from build123d import *

# Parameters (mm, degrees)
F0_W           = 304.8
F0_H           = 25.4
F1_DEPTH       = 101.6
F3_DEPTH       = 101.6
F5_D           = 10.0838
F5_CSINK_D     = 19.8374
F5_CSINK_ANGLE = 82
F7_D           = 13.49248
F8_SIZE        = 9.525
F9_SIZE        = 9.525


with BuildPart() as f1:
    # F0 (on Front) → F1 (new body, symmetric)
    with BuildSketch(Plane.XZ):
        Rectangle(F0_W, F0_H)
    extrude(amount=F1_DEPTH, both=True)

    # F2 (on Right) → F3 (join, symmetric)
    with BuildSketch(Plane.YZ):
        with BuildLine():
            Line((-82.55, 19.05), (-82.55, 12.7))
            Line((-82.55, 12.7), (-6.35, 12.7))
            Line((-6.35, 12.7), (-6.35, 88.9))
            Line((-6.35, 88.9), (-12.7, 88.9))
            ThreePointArc((-12.7, 88.9), (-14.9450640303, 87.9700640303), (-15.875, 85.725))
            Line((-15.875, 85.725), (-15.875, 28.575))
            ThreePointArc((-15.875, 28.575), (-17.7348719395, 24.0848719395), (-22.225, 22.225))
            Line((-22.225, 22.225), (-79.375, 22.225))
            ThreePointArc((-79.375, 22.225), (-81.6200640303, 21.2950640303), (-82.55, 19.05))
        make_face()
        with BuildLine():
            Line((6.35, 88.9), (6.35, 12.7))
            Line((6.35, 12.7), (82.55, 12.7))
            Line((82.55, 12.7), (82.55, 19.05))
            ThreePointArc((82.55, 19.05), (81.6200640303, 21.2950640303), (79.375, 22.225))
            Line((79.375, 22.225), (22.225, 22.225))
            ThreePointArc((22.225, 22.225), (17.7348719395, 24.0848719395), (15.875, 28.575))
            Line((15.875, 28.575), (15.875, 85.725))
            ThreePointArc((15.875, 85.725), (14.9450640303, 87.9700640303), (12.7, 88.9))
            Line((12.7, 88.9), (6.35, 88.9))
        make_face()
    extrude(amount=F3_DEPTH, both=True)

    # F5 (through all)
    with Locations(Plane(origin=(0, 0, -12.7), x_dir=(1, 0, 0), z_dir=(0, 0, -1))):
        with Locations((-76.2, 50.8), (76.2, 50.8), (76.2, -50.8), (-76.2, -50.8)):
            CounterSinkHole(F5_D / 2, F5_CSINK_D / 2, counter_sink_angle=F5_CSINK_ANGLE)

    # F7 (through all)
    with Locations(Plane.XZ.offset(15.875)):
        with Locations((-63.5, 60.325), (63.5, 60.325)):
            Hole(F7_D / 2)

    # F8
    f8_edges = [f1.edges().sort_by_distance(p)[0] for p in [
        (152.4, 0, -12.7),
    ]]
    chamfer(f8_edges, length=F8_SIZE)

    # F9
    f9_edges = [f1.edges().sort_by_distance(p)[0] for p in [
        (-152.4, 0, -12.7),
    ]]
    chamfer(f9_edges, length=F9_SIZE)


solid = f1.part
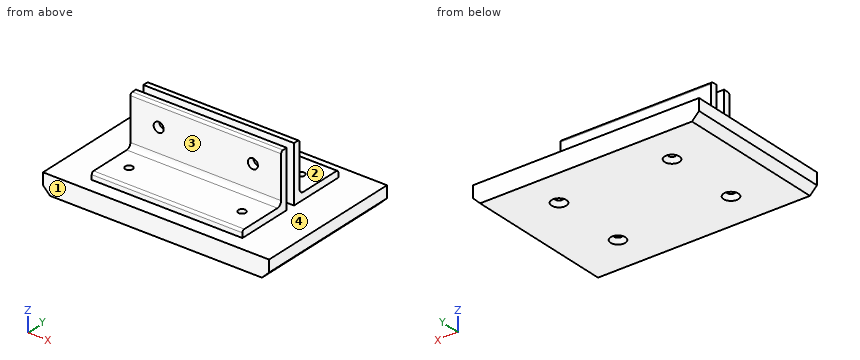
The listing builds one solid part. Answer for the finished solid, in the listing's coordinates (mm). Face numbers are marked on the shaded views. A direction names the side the tool comes from. Coordinates: 2 decimals unless noted, no trailing zeros. Loops run counter-clockwise (first coordinate to the right, second up) from the corner with the lowest first, then second, coordinate; pieces in that order, holes last.
1) Flat-ended cylindrical pins translate along their axes: pin 1 Ø17.5 at (x, z) = (63.5, 60.325) entering from -Y (3 decimals); pin 2 Ø1 at (y, z) = (9.5, 50.5) entering from -X; pin 3 Ø1.9 at (x, z) = (22, 16) entering from -Y. Find the tip coordinate at first contact, or state that the pin passes through.
2) Find section B-B on z = 48. Write down the section's boundary in (x, y) (3 decimals), then the cut area to 3 significant figures.
3) Find the intervals of material crossed by L1, parallel to X at y = 50, z = 9; L2, parallel to Y at x = -76, z = 4; L3, parallel to Y at x = 39.5, z = 19.5, in increasing order.
4) Find section A-A on x = -76.2. Give the number of separate pieces and of enclosed holes in the cut face, then the cut area to 3 significant figures.
5) A tool of negligible diameter and unlimited length cuts with its end or side. For the marked faces 1, 2, 3 and 4, from which of +Z, -Z, +X, -X, +Y, -Y can it reach the whole face along a straight path? Write none if from no direction.
6) Find section C-C on y = 50.8. Write down the section's boundary in (x, z) (3 decimals), then the cut area to 3 significant figures.
7) Find section D-D on y = -72.5. Write down the section's boundary in (x, z) (3 decimals), then the cut area to 3 significant figures.
Values:
1. pin 1: stops at y = -15.875
1. pin 2: stops at x = -101.6
1. pin 3: stops at y = -82.55
2. outline: (-101.6, -15.875) - (101.6, -15.875) - (101.6, -6.35) - (-101.6, -6.35) - close; (-101.6, 6.35) - (101.6, 6.35) - (101.6, 15.875) - (-101.6, 15.875) - close
2. area: 3,870 mm2
3. L1: x = -152.4 to -81.18, -71.22 to 71.22, 81.18 to 152.4
3. L2: y = -101.6 to -55.84, -45.76 to 45.76, 55.84 to 101.6
3. L3: y = -82.52 to -6.35, 6.35 to 82.52
4. separate pieces: 3
4. enclosed holes: 0
4. area: 7,130 mm2
5. face 1: +Z, -Z, +X, -X, -Y
5. face 2: +Z, +X, -X, +Y
5. face 3: +Z, +X, -X, -Y
5. face 4: +Z
6. outline: (-152.4, -3.175) - (-142.875, -12.7) - (-86.119, -12.7) - (-81.242, -7.09) - (-81.242, 22.225) - (-101.6, 22.225) - (-101.6, 12.7) - (-152.4, 12.7) - close; (-71.158, -7.09) - (-66.281, -12.7) - (66.281, -12.7) - (71.158, -7.09) - (71.158, 22.225) - (-71.158, 22.225) - close; (81.242, -7.09) - (86.119, -12.7) - (142.875, -12.7) - (152.4, -3.175) - (152.4, 12.7) - (101.6, 12.7) - (101.6, 22.225) - (81.242, 22.225) - close
6. area: 8,830 mm2
7. outline: (-152.4, -3.175) - (-142.875, -12.7) - (142.875, -12.7) - (152.4, -3.175) - (152.4, 12.7) - (101.6, 12.7) - (101.6, 22.225) - (-101.6, 22.225) - (-101.6, 12.7) - (-152.4, 12.7) - close
7. area: 9,590 mm2
